Check sheet for the modelled part. Datum: model origin and axes. Units: mm. Round coordinates to 2 decimals unless told otherwise and drop trailing zeros. Write each loop counter-clockwise with the first axis right and the second up, starting at its lowest first coordinate (ties: lowest second). Pieces come first, ordered by that corner, then holes.
Item 1: Material ranges on line 1 along Y through (x, z) = (-15, 2.8); line 2 along X through (y, z) = (-1, 2.8); line 3 along Y through (x, z) = (1.5, 0.45), recorded low to high.
Item 2: Section check A-A, the plane y = 0. Record the cut outline in (x, z).
Item 3: Release check for a two-part mould opening along X. For faces 1 (the flat face through (-22.5, 0, 3)), 2 (the cylindrical face through (-16.669, -0.526, 2.398)), 3 (the flat face through (22.5, 0, 3)) record: pulls with the +X half, pulls with the -X half, needs draft (parallel to the pull), parting line crosses it, or undercut.
Item 4: Depth check by flat-ended pin: pin 1 (6 mm diameter, centred on x = -1, y = 1, fed in from +Z); pin 2 (4 mm diameter, centred on x = 15, y = 0, fed in from -Z). Enter the tip coordinate at first touch or a pass-through.
Item 5: Section check B-B, the plane x = -15. Record the cut outline in (y, z).
Item 6: Section check C-C, the plane z = 2.85. Record the cut outline in (x, y).
Item 7: Section check D-D, the plane x = -8. Record the cut outline in (y, z), plus the area to 3 significant figures.
from build123d import *

# Parameters (mm, degrees)
F0_W           = 45
F0_H           = 12
F1_DEPTH       = 4
F2_D           = 3.5
F2_CSINK_D     = 5
F2_CSINK_ANGLE = 90
F3_R           = 1.5
F4_T1_DEPTH    = 9
F4_T4_ANGLE    = 90
F4_T6_ANGLE    = 90
F4_T8_ANGLE    = 90
F4_T10_ANGLE   = 90


# Not quite as in the source:
# - a fillet or chamfer that OpenCascade refuses, or shapes differently, is made with other operations: its cross-section is extruded or revolved along the edge and cut away or added


with BuildPart() as f1:
    # F0 (on Top) → F1 (new body)
    with BuildSketch(Plane.XY):
        Rectangle(F0_W, F0_H)
    extrude(amount=F1_DEPTH)

    # F2 (through all)
    with Locations(Plane(origin=(0, 0, 0), x_dir=(1, 0, 0), z_dir=(0, 0, -1))):
        with Locations((-15, 0), (0, 0), (15, 0)):
            CounterSinkHole(F2_D / 2, F2_CSINK_D / 2, counter_sink_angle=F2_CSINK_ANGLE)

    # F3
    f3_edges = [f1.edges().sort_by_distance(p)[0] for p in [
        (0, -6, 0),
        (-22.5, 0, 0),
        (0, 6, 0),
        (22.5, 0, 0),
    ]]
    fillet(f3_edges, radius=F3_R)

    # F4: fillet of radius 2 on 4 edges, made by hand

    # F4_s2 → F4_t1 (cut)
    with BuildSketch(Plane.XY):
        with BuildLine():
            ThreePointArc((22.5, -4), (21.9142135624, -5.4142135624), (20.5, -6))
            Line((20.5, -6), (22.5, -6))
            Line((22.5, -6), (22.5, -4))
        make_face()
        with BuildLine():
            ThreePointArc((20.5, 6), (21.9142135624, 5.4142135624), (22.5, 4))
            Line((22.5, 4), (22.5, 6))
            Line((22.5, 6), (20.5, 6))
        make_face()
        with BuildLine():
            ThreePointArc((-22.5, -4), (-21.9142135624, -5.4142135624), (-20.5, -6))
            Line((-20.5, -6), (-22.5, -6))
            Line((-22.5, -6), (-22.5, -4))
        make_face()
        with BuildLine():
            ThreePointArc((-20.5, 6), (-21.9142135624, 5.4142135624), (-22.5, 4))
            Line((-22.5, 4), (-22.5, 6))
            Line((-22.5, 6), (-20.5, 6))
        make_face()
    extrude(amount=F4_T1_DEPTH, mode=Mode.SUBTRACT)

    # F4_s3 → F4_t4 (revolve, cut)
    with BuildSketch(Plane.XZ.offset(-4)):
        with BuildLine():
            ThreePointArc((-21, 0), (-22.0606601718, 0.4393398282), (-22.5, 1.5))
            Line((-22.5, 1.5), (-22.5, 0))
            Line((-22.5, 0), (-21, 0))
        make_face()
    revolve(axis=Axis((-20.5, 4, 0), (0, 0, -1)), revolution_arc=F4_T4_ANGLE, mode=Mode.SUBTRACT)

    # F4_s5 → F4_t6 (revolve, cut)
    with BuildSketch(Plane.YZ.offset(-20.5)):
        with BuildLine():
            ThreePointArc((-4.5, 0), (-5.5606601718, 0.4393398282), (-6, 1.5))
            Line((-6, 1.5), (-6, 0))
            Line((-6, 0), (-4.5, 0))
        make_face()
    revolve(axis=Axis((-20.5, -4, 0), (0, 0, -1)), revolution_arc=F4_T6_ANGLE, mode=Mode.SUBTRACT)

    # F4_s7 → F4_t8 (revolve, cut)
    with BuildSketch(Plane.YZ.offset(20.5)):
        with BuildLine():
            ThreePointArc((4.5, 0), (5.5606601718, 0.4393398282), (6, 1.5))
            Line((6, 1.5), (6, 0))
            Line((6, 0), (4.5, 0))
        make_face()
    revolve(axis=Axis((20.5, 4, 0), (0, 0, -1)), revolution_arc=F4_T8_ANGLE, mode=Mode.SUBTRACT)

    # F4_s9 → F4_t10 (revolve, cut)
    with BuildSketch(Plane.XZ.offset(4)):
        with BuildLine():
            ThreePointArc((21, 0), (22.0606601718, 0.4393398282), (22.5, 1.5))
            Line((22.5, 1.5), (22.5, 0))
            Line((22.5, 0), (21, 0))
        make_face()
    revolve(axis=Axis((20.5, -4, 0), (0, 0, -1)), revolution_arc=F4_T10_ANGLE, mode=Mode.SUBTRACT)


solid = f1.part
Values found:
1. line 1: y = -6 to -1.75, 1.75 to 6
1. line 2: x = -22.5 to -16.44, -13.56 to -1.44, 1.44 to 13.56, 16.44 to 22.5
1. line 3: y = -5.57 to -1.4, 1.4 to 5.57
2. outline: (-22.5, 1.5) arc R1.5 ccw to (-21, 0) - (-17.5, 0) - (-16.75, 0.75) - (-16.75, 4) - (-22.5, 4) - close; (-13.25, 0.75) - (-12.5, 0) - (-2.5, 0) - (-1.75, 0.75) - (-1.75, 4) - (-13.25, 4) - close; (1.75, 0.75) - (2.5, 0) - (12.5, 0) - (13.25, 0.75) - (13.25, 4) - (1.75, 4) - close; (16.75, 0.75) - (17.5, 0) - (21, 0) arc R1.5 ccw to (22.5, 1.5) - (22.5, 4) - (16.75, 4) - close
3. face 1: pulls with the -X half
3. face 2: undercut
3. face 3: pulls with the +X half
4. pin 1: stops at z = 4
4. pin 2: stops at z = 0.5
5. outline: (-6, 1.5) arc R1.5 ccw to (-4.5, 0) - (-2.5, 0) - (-1.75, 0.75) - (-1.75, 4) - (-6, 4) - close; (1.75, 0.75) - (2.5, 0) - (4.5, 0) arc R1.5 ccw to (6, 1.5) - (6, 4) - (1.75, 4) - close
6. outline: (-22.5, -4) arc R2 ccw to (-20.5, -6) - (20.5, -6) arc R2 ccw to (22.5, -4) - (22.5, 4) arc R2 ccw to (20.5, 6) - (-20.5, 6) arc R2 ccw to (-22.5, 4) - close; hole circle Ø3.5 at (-15, 0); hole circle Ø3.5 at (0, 0); hole circle Ø3.5 at (15, 0)
7. outline: (-6, 1.5) arc R1.5 ccw to (-4.5, 0) - (4.5, 0) arc R1.5 ccw to (6, 1.5) - (6, 4) - (-6, 4) - close
7. area: 47.0 mm2
